Can you work these out from the model? Positions are in its coordinate system, mm. Round coordinates to 2 decimals unless told otherwise and drop trailing zeros. Loops run counter-clockwise (first coordinate to the right, second up) from the corner with the lowest first, then second, coordinate; pieces in that order, holes last. Notation, with made-up numbers: (7, 43) -> (56, 43) arc R16 ccw to (56, 47) -> close; hole circle Ø4 at (45.25, -33.75). An arc over 180 degrees is marked (long way). Answer as a JSON object with one key per item and string values.
```python
from build123d import *

# Parameters (mm, degrees)
IZIM1_R                     = 8
IZIM1_R_2                   = 2.1
IZIM1_R_3                   = 1.25
Y_KSEKLIK_EKSTR_ZYON1_DEPTH = 10


with BuildPart() as part:
    # Çizim1 → Yükseklik-Ekstrüzyon1 (new body)
    with BuildSketch(Plane.XY):
        with BuildLine():
            Line((-35, 17.5), (35, 17.5))
            ThreePointArc((35, 17.5), (52.5, 0), (35, -17.5))
            Line((35, -17.5), (-35, -17.5))
            ThreePointArc((-35, -17.5), (-52.5, 0), (-35, 17.5))
        make_face()
        Circle(IZIM1_R, mode=Mode.SUBTRACT)
        with Locations((-35, 0)):
            Circle(IZIM1_R_2, mode=Mode.SUBTRACT)
        with Locations((0, 11)):
            Circle(IZIM1_R_3, mode=Mode.SUBTRACT)
        with Locations((9.526279442, 5.5)):
            Circle(IZIM1_R_3, mode=Mode.SUBTRACT)
        with Locations((9.526279442, -5.5)):
            Circle(IZIM1_R_3, mode=Mode.SUBTRACT)
        with Locations((0, -11)):
            Circle(IZIM1_R_3, mode=Mode.SUBTRACT)
        with Locations((-9.526279442, -5.5)):
            Circle(IZIM1_R_3, mode=Mode.SUBTRACT)
        with Locations((-9.526279442, 5.5)):
            Circle(IZIM1_R_3, mode=Mode.SUBTRACT)
        with Locations((35, 0)):
            Circle(IZIM1_R_2, mode=Mode.SUBTRACT)
    extrude(amount=Y_KSEKLIK_EKSTR_ZYON1_DEPTH)


solid = part.part
```
Q1. I want a section at C-C, the plane z = 4.5. Give the number of separate pieces and of enclosed holes in the cut face, then the cut area to 3 significant figures.
Determined:
{"separate pieces": "1", "enclosed holes": "9", "area": "3,150 mm²"}
Q2. If I drill on L1, parallel to Y at x = 0, z = 7.25; L2, parallel to X at y = 5, z = 2.75 (1 decimal); L3, parallel to Y at x = -35, z = 2.5, over which ranges is the centre line in solid material (lowest first)? Write a range as [from, to].
Determined:
{"L1": "[-17.5, -12.25], [-9.75, -8], [8, 9.75], [12.25, 17.5]", "L2": "[-51.8, -10.7], [-8.4, -6.2], [6.2, 8.4], [10.7, 51.8]", "L3": "[-17.5, -2.1], [2.1, 17.5]"}
Q3. I want a section at B-B, the plane y = -11. Write out the boundary of the cut face in (x, z).
Determined:
{"outline": "(-48.61, 0) -> (-1.25, 0) -> (-1.25, 10) -> (-48.61, 10) -> close; (1.25, 0) -> (48.61, 0) -> (48.61, 10) -> (1.25, 10) -> close"}
Q4. I want a section at D-D, the plane y = -5.5. Write out the boundary of the cut face in (x, z), then the cut area to 3 significant figures.
Determined:
{"outline": "(-51.61, 0) -> (-10.78, 0) -> (-10.78, 10) -> (-51.61, 10) -> close; (-8.28, 0) -> (-5.81, 0) -> (-5.81, 10) -> (-8.28, 10) -> close; (5.81, 0) -> (8.28, 0) -> (8.28, 10) -> (5.81, 10) -> close; (10.78, 0) -> (51.61, 0) -> (51.61, 10) -> (10.78, 10) -> close", "area": "866 mm²"}
Q5. We'd pull the mould along Y, two halves only. Please class faces 1 (the cylindrical face through (-52.496, -0.385, 4.93)), 2 (the cylindrical face through (10.68, -5.98, 4.93)), 3 (the flat face through (12, 0, 10)): pulls with the +Y half, pulls with the -Y half, needs draft (parallel to the pull), parting line crosses it, or undercut.
Determined:
{"face 1": "parting line crosses it", "face 2": "undercut", "face 3": "needs draft"}
Q6. I'm going to push flat-ended pins straight in: pin 1 (1 mm diameter, centred on y = 10.5, z = 8, fed in from +X); pin 2 (4 mm diameter, centred on y = -11.5, z = 4, fed in from -X); pin 3 (1 mm diameter, centred on y = -4.5, z = 1.5, fed in from +X). Where does each tip first touch, or does it pass through?
Determined:
{"pin 1": "x = 49.36", "pin 2": "x = -49.7", "pin 3": "x = 52.04"}
Q7. I want a section at A-A, the plane y = 0. Write out the boundary of the cut face in (x, z).
Determined:
{"outline": "(-52.5, 0) -> (-37.1, 0) -> (-37.1, 10) -> (-52.5, 10) -> close; (-32.9, 0) -> (-8, 0) -> (-8, 10) -> (-32.9, 10) -> close; (8, 0) -> (32.9, 0) -> (32.9, 10) -> (8, 10) -> close; (37.1, 0) -> (52.5, 0) -> (52.5, 10) -> (37.1, 10) -> close"}
